from build123d import *

# Parameters (mm, degrees)
F0_R     = 46.410682
F0_R_2   = 3.651099
F0_R_3   = 3.351621
F0_R_4   = 34.602582
F0_R_5   = 3.373279
F1_DEPTH = 5.08
F0_R_6   = 4.231249
F0_R_7   = 3.946303
F2_DEPTH = 3.81
F3_DEPTH = 16.764
F4_DEPTH = 16.764
F5_R     = 4.263251
F6_DEPTH = 22.606


with BuildPart() as f1:
    # F0 (on Front) → F1 (new body)
    with BuildSketch(Plane.XZ):
        Circle(F0_R)
        with Locations((0, -40.69474)):
            Circle(F0_R_2, mode=Mode.SUBTRACT)
        with Locations((-40.69474, 0)):
            Circle(F0_R_3, mode=Mode.SUBTRACT)
        Circle(F0_R_4, mode=Mode.SUBTRACT)
        with Locations((26.899913, 30.841293)):
            Circle(F0_R_5, mode=Mode.SUBTRACT)
    extrude(amount=F1_DEPTH)

    # F0 (on Front) → F2 (join)
    with BuildSketch(Plane.XZ):
        Circle(F0_R_4)
        with Locations((6.010604, -5.222328)):
            Circle(F0_R_6, mode=Mode.SUBTRACT)
        with Locations((10.543191, 14.681638)):
            Circle(F0_R_7, mode=Mode.SUBTRACT)
    extrude(amount=F2_DEPTH)

    # F0 (on Front) → F3 (join)
    with BuildSketch(Plane.XZ):
        with Locations((-40.69474, 0)):
            Circle(F0_R_3)
    extrude(amount=F3_DEPTH)

    # F0 (on Front) → F4 (join)
    with BuildSketch(Plane.XZ):
        with Locations((0, -40.69474)):
            Circle(F0_R_2)
        with Locations((26.899913, 30.841293)):
            Circle(F0_R_5)
    extrude(amount=F4_DEPTH)

    # F5 (on Front) → F6 (join)
    with BuildSketch(Plane.XZ):
        with Locations((-9.77318, -20.470712)):
            Circle(F5_R)
    extrude(amount=-F6_DEPTH)


solid = f1.part
Part model, mm, in its own coordinate system. A direction names the side the tool comes from. Give positions to 0.01 mm unless a question says otherwise; leave off trailing zeros. Write each loop counter-clockwise with the first axis right and the second up, starting at its lowest first coordinate (ties: lowest second). Pieces come first, ordered by that corner, then holes.
1) Pin check, flat tips, straight feed: pin 1 (21 mm diameter, centred on x = 1.5, z = -7.5, fed in from -Y); pin 2 (5 mm diameter, centred on y = 12.5, z = -24, fed in from +X); pin 3 (8 mm diameter, centred on x = 35, z = 5, fed in from -Y). Stop position of each tip, or through.
Resolved:
pin 1: stops at y = -3.81
pin 2: stops at x = -5.64
pin 3: stops at y = -5.08
2) Two-plate mould, pull along X, no slides. Class faces 4 (the face through (44.268, -2.504, 13.941)), 5 (the face through (27, -16.764, 31)), 6 (the face through (33.005, -4.436, 10.394)), 7 (the face through (0, -3.81, 0)): released by +X, released by -X, zero draft, split by the parting line, or undercut.
Resolved:
face 4: split by the parting line
face 5: zero draft
face 6: undercut
face 7: undercut
3) Cut at A-A on x = 5. Write the cut outline in (y, z), then the cut area to 3 significant figures.
Resolved:
outline: (-5.08, -46.14) - (0, -46.14) - (0, -9.33) - (-3.81, -9.33) - (-3.81, -34.24) - (-5.08, -34.24) - close; (-5.08, 34.24) - (-3.81, 34.24) - (-3.81, -1.11) - (0, -1.11) - (0, 46.14) - (-5.08, 46.14) - close
area: 351 mm2
4) Cut at B-B on z = -28.5. Write the cut outline in (x, y), then the cut area to 3 significant figures.
Resolved:
outline: (-36.63, -5.08) - (-19.62, -5.08) - (-19.62, -3.81) - (19.62, -3.81) - (19.62, -5.08) - (36.63, -5.08) - (36.63, 0) - (-36.63, 0) - close
area: 322 mm2
5) Cut at C-C on y = -8. Write the cut outline in (x, z).
Resolved:
outline: circle Ø6.7 at (-40.69, 0); circle Ø7.3 at (0, -40.69); circle Ø6.75 at (26.9, 30.84)
6) Probe L1, parallel to Z at x = 0, y = -4; L2, parallel to Y at x = 15, z = 40; L3, parallel to Z at x = 8.5, y = -1.5. List the from-to ranges inside material, lowest first.
Resolved:
L1: z = -46.41 to -34.6, 34.6 to 46.41
L2: y = -5.08 to 0
L3: z = -45.63 to -8.64, -1.8 to 11.31, 18.06 to 45.63
7) Cut at D-D on y = 20. Write the cut outline in (x, z), then the cut area to 3 significant figures.
Resolved:
outline: circle Ø8.53 at (-9.77, -20.47)
area: 57.1 mm2
8) Which spindle directions (+Z, -Z, +X, -X, +Y, -Y) get a long thin tool onto all of the face, cutting with end or side? Do faces 1 (the face through (-7.806, 11.145, -24.253)), 2 (the face through (-41, -16.764, 0)), 3 (the face through (-38.893, -10.84, 2.826)). Say none if no direction does.
Resolved:
face 1: +Y
face 2: +Z, -Z, +X, -X, -Y
face 3: -Y
